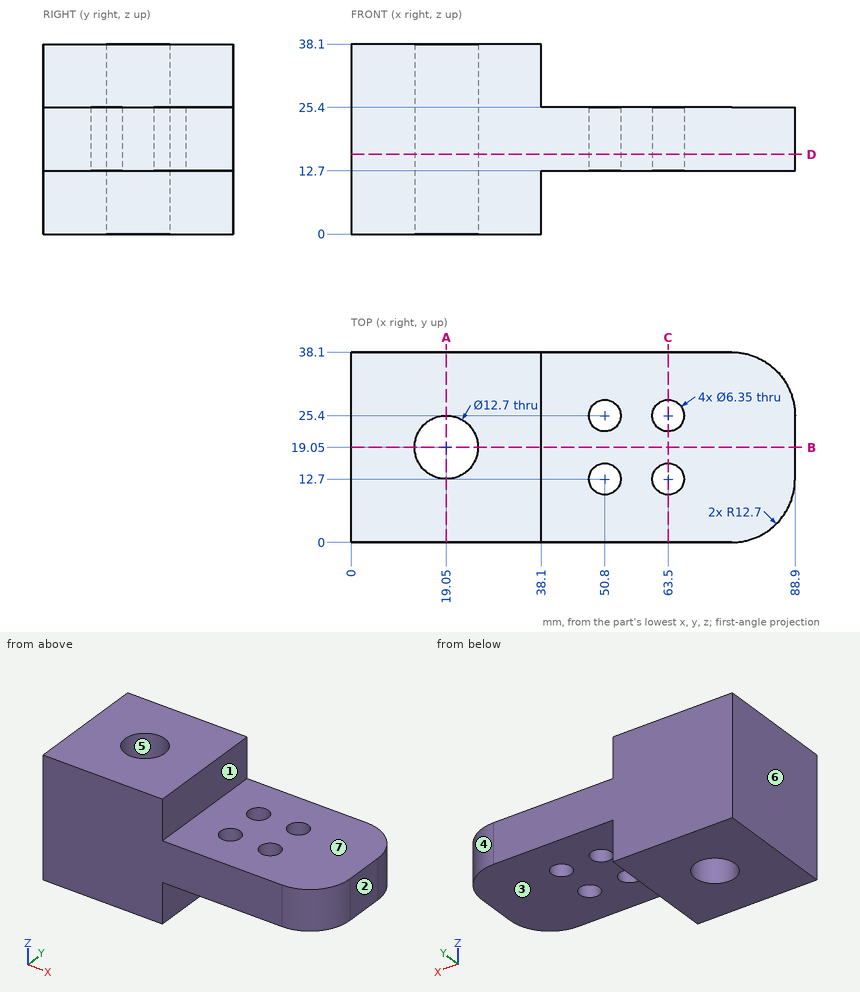
Check sheet for the drawn part. Datum: minimum x, y, z corner. Units: mm. A direction names the side the tool comes from. Give positions to 0.01 mm unless a question says otherwise; leave off trailing zeros. Loops run counter-clockwise (first coordinate to the right, second up) from the corner with the lowest first, then second, coordinate; pieces in that order, holes last.
1) Sectioned sample at D-D, the plane z = 16. Enter the section's corners in (x, y) (3 decimals).
2) Draft check along X on the marked faces 4, 5, 6 and 7. Enter one of: pulls with the +X half, pulls with the -X half, needs draft (parallel to the pull), parting line crosses it, or undercut.
3) Thickness scan on line 1 along Y through (x, z) = (50.8, 16) (3 decimals); line 2 along X through (y, z) = (19, 16); line 3 along Y through (x, z) = (63, 19). Record the ranges inside material, lowest first.
4) Sectioned sample at B-B, the plane y = 19.05. Enter the section's corners in (x, z).
5) Sectioned sample at A-A, the plane x = 19.05. Enter the section's corners in (y, z).
6) Depth check by flat-ended pin: pin 1 Ø8.5 at (x, y) = (50.8, 25.4) entering from -Z; pin 2 Ø11.5 at (x, y) = (19.05, 19.05) entering from +Z; pin 3 Ø11.5 at (x, y) = (51, 28.5) entering from +Z; pin 4 Ø3 at (y, z) = (33.5, 30.5) entering from +X. Enter the tip coordinate at first touch or a pass-through.
7) Sectioned sample at C-C, the plane x = 63.5. Enter the section's corners in (y, z) (3 decimals), then the cut area to 3 significant figures.
8) Set-up check for the marked faces 1, 2 and 3: record each of +Z, -Z, +X, -X, +Y, -Y from which the full face is reachable in a straight line by a thin tool's end or side.
Answers:
1. outline: (0, 0) - (76.2, 0) arc R12.7 ccw to (88.9, 12.7) - (88.9, 25.4) arc R12.7 ccw to (76.2, 38.1) - (0, 38.1) - close; hole circle Ø12.7 at (19.05, 19.05); hole circle Ø6.35 at (50.8, 12.7); hole circle Ø6.35 at (50.8, 25.4); hole circle Ø6.35 at (63.5, 12.7); hole circle Ø6.35 at (63.5, 25.4)
2. face 4: pulls with the +X half
2. face 5: undercut
2. face 6: pulls with the -X half
2. face 7: needs draft
3. line 1: y = 0 to 9.525, 15.875 to 22.225, 28.575 to 38.1
3. line 2: x = 0 to 12.7, 25.4 to 88.9
3. line 3: y = 0 to 9.56, 15.84 to 22.26, 28.54 to 38.1
4. outline: (0, 0) - (12.7, 0) - (12.7, 38.1) - (0, 38.1) - close; (25.4, 0) - (38.1, 0) - (38.1, 12.7) - (88.9, 12.7) - (88.9, 25.4) - (38.1, 25.4) - (38.1, 38.1) - (25.4, 38.1) - close
5. outline: (0, 0) - (12.7, 0) - (12.7, 38.1) - (0, 38.1) - close; (25.4, 0) - (38.1, 0) - (38.1, 38.1) - (25.4, 38.1) - close
6. pin 1: stops at z = 12.7
6. pin 2: passes through
6. pin 3: stops at z = 25.4
6. pin 4: stops at x = 38.1
7. outline: (0, 12.7) - (9.525, 12.7) - (9.525, 25.4) - (0, 25.4) - close; (15.875, 12.7) - (22.225, 12.7) - (22.225, 25.4) - (15.875, 25.4) - close; (28.575, 12.7) - (38.1, 12.7) - (38.1, 25.4) - (28.575, 25.4) - close
7. area: 323 mm2
8. face 1: +Z, +X, +Y, -Y
8. face 2: +Z, -Z, +X, +Y, -Y
8. face 3: -Z, +X, +Y, -Y
